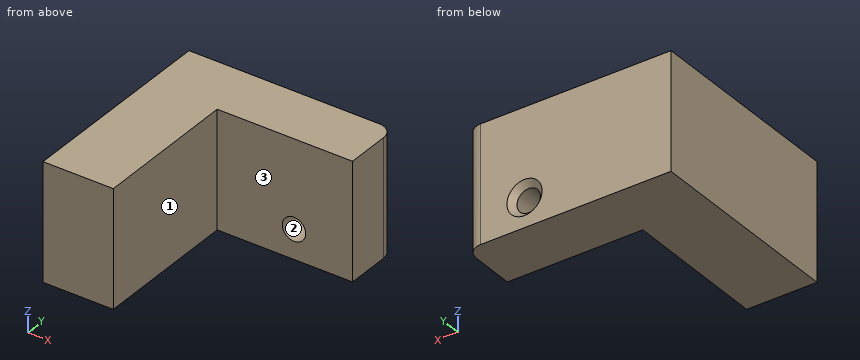
```python
from build123d import *

# Parameters (mm, degrees)
F1_DEPTH       = 20
F3_D           = 4
F3_CSINK_D     = 6
F3_CSINK_ANGLE = 90
F4_R           = 2.5


with BuildPart() as f1:
    # F0 (on Top) → F1 (new body)
    with BuildSketch(Plane.XY):
        Polygon((-4.108734, 30.537107), (-4.213165, -4.462893), (7.786835, -4.462893), (7.786835, 20.537107), (30.891266, 20.537107), (30.891266, 30.537107), align=None)
    extrude(amount=F1_DEPTH)

    # F3 (through all)
    with Locations(Plane(origin=(0, 30.537107, 0), x_dir=(-1, 0, 0), z_dir=(0, 1, 0))):
        with Locations((-20.891266, 5)):
            CounterSinkHole(F3_D / 2, F3_CSINK_D / 2, counter_sink_angle=F3_CSINK_ANGLE)

    # F4
    f4_edges = [f1.edges().sort_by_distance(p)[0] for p in [
        (30.891266, 30.537107, 10),
    ]]
    fillet(f4_edges, radius=F4_R)


solid = f1.part
```
CAD build for the part. Positions are in the model's coordinates, mm. Face numbers are marked on the shaded views. Coordinates: 2 decimals unless noted, no trailing zeros. Write each loop counter-clockwise with the first axis right and the second up, starting at its lowest first coordinate (ties: lowest second). Pieces come first, ordered by that corner, then holes.
(1) Cut at A-A, the plane z = 5. List the corners of the cut face in (x, y), and give its area (3 significant figures).
(2) Two-plate mould, pull along X, no slides. Class the marked faces 1, 2 and 3: +X half, -X half, draft (parallel to the pull), parting line (faces both ways), or undercut.
(3) Cut at B-B, the plane z = 8.5. List the corners of the cut face in (x, y).
(4) Flat gauge pins, fed straight in: pin 1 (3.5 mm diameter, centred on x = 20.89, z = 5, fed in from +Y); pin 2 (3 mm diameter, centred on x = 22, z = 3, fed in from -Y); pin 3 (3 mm diameter, centred on y = 9.5, z = 17, fed in from -X). Where does each tip first touch, or does it go through?
(5) Drill centre lines: probe 1 along X at (y, z) = (27.75, 5); probe 2 along Y at (x, z) = (12.5, 17.5); probe 3 along X at (y, z) = (-1, 7.5). Where is each one in solid material? Low to high.
(6) Cut at C-C, the plane y = 27.5. List the corners of the cut face in (x, z).
(7) Cut at D-D, the plane x = 14. List the corners of the cut face in (y, z), and give its area (3 significant figures).
Geometry says:
1. outline: (-4.21, -4.46) - (7.79, -4.46) - (7.79, 20.54) - (18.89, 20.54) - (18.89, 29.54) - (17.89, 30.54) - (-4.11, 30.54) - close; (22.89, 20.54) - (30.89, 20.54) - (30.89, 28.04) arc R2.5 ccw to (28.39, 30.54) - (23.89, 30.54) - (22.89, 29.54) - close
1. area: 607 mm2
2. face 1: +X half
2. face 2: undercut
2. face 3: draft
3. outline: (-4.21, -4.46) - (7.79, -4.46) - (7.79, 20.54) - (30.89, 20.54) - (30.89, 28.04) arc R2.5 ccw to (28.39, 30.54) - (-4.11, 30.54) - close
4. pin 1: passes through
4. pin 2: stops at y = 20.54
4. pin 3: stops at x = -4.18
5. probe 1: x = -4.12 to 18.89, 22.89 to 30.89
5. probe 2: y = 20.54 to 30.54
5. probe 3: x = -4.2 to 7.79
6. outline: (-4.12, 0) - (30.89, 0) - (30.89, 20) - (-4.12, 20) - close; hole circle Ø4 at (20.89, 5)
7. outline: (20.54, 0) - (30.54, 0) - (30.54, 20) - (20.54, 20) - close
7. area: 200 mm2
